from build123d import *

# Parameters (mm, degrees)
CROQUIS1_R              = 4.98
SALIENTE_EXTRUIR1_DEPTH = 4
CROQUIS2_R              = 4.98
SALIENTE_EXTRUIR2_DEPTH = 4
CORTAR_EXTRUIR1_DEPTH   = 12.160680983


with BuildPart() as part:
    # Croquis1 → Saliente-Extruir1 (new body)
    with BuildSketch(Plane(origin=(0, 0, 0), x_dir=(1, 0, 0), z_dir=(0, 1, 0))):
        with Locations(Location((1, 0, 0), (0, 0, 270))):
            Circle(CROQUIS1_R)
    extrude(amount=SALIENTE_EXTRUIR1_DEPTH)

    # Croquis2 → Saliente-Extruir2 (add)
    with BuildSketch(Plane(origin=(0, 4, 0), x_dir=(1, 0, 0), z_dir=(0, 1, 0))):
        with Locations(Location((-1, 0, 0), (0, 0, 78.416067345))):
            Circle(CROQUIS2_R)
    extrude(amount=SALIENTE_EXTRUIR2_DEPTH)

    # Croquis3 → Cortar-Extruir1 (cut, through all)
    with BuildSketch(Plane(origin=(0, 0, 0), x_dir=(1, 0, 0), z_dir=(0, 1, 0))):
        with BuildLine():
            Line((-1.559847749, 2.65), (1.559847749, 2.65))
            ThreePointArc((1.559847749, 2.65), (0, -3.075), (-1.559847749, 2.65))
        make_face()
    extrude(amount=CORTAR_EXTRUIR1_DEPTH, mode=Mode.SUBTRACT)


solid = part.part
Input: part model. Units: mm. Frame: model coordinates. A direction names the side the tool comes from. Round coordinates to 2 decimals unless told otherwise and drop trailing zeros. Loops run counter-clockwise (first coordinate to the right, second up) from the corner with the lowest first, then second, coordinate; pieces in that order, holes last. Notation, with made-up numbers: M 81.5,23 L 89.5,23 A13 cw 89.5,39 Z; hole C -29,74 d8. An arc over 180 degrees is marked long. Answer as CSV lines item,"result". Start each with the question number.
(1) Section B-B, the plane z = 1.5. Output: boundary loops of the cut face in (x, y), plus the area to 3 significant figures.
(2) Reachability of faces 1 (the flat face through (4.3, 4, 0.3)), 2 (the cylindrical face through (2.5, 1.97, 4.75)), 3 (the flat face through (-4.4, 4, 0.1)) from +Z, -Z, +X, -X, +Y, -Y: full face, straight path, thin tool, end or side. Return the list, or none.
(3) Section A-A, the plane x = -2.25. Output: boundary loops of the cut face in (y, z), plus the area to 3 significant figures.
(4) Draft query along Z for faces 4 (the flat face through (0, 4, -2.65)), 5 (the cylindrical face through (-1.512, 5.972, -4.954)), 6 (the flat face through (-3.3, 8, -0.4)). Return one class per face: released by +Z, released by -Z, zero draft, split by the parting line, or undercut.
(5) Section D-D, the plane x = 4.5. Output: boundary loops of the cut face in (y, z), plus the area to 3 significant figures.
(6) First-contact query: pin 1 (5 mm diameter, centred on x = 0, z = 0, fed in from -Y); pin 2 (1.5 mm diameter, centred on y = 3.5, z = 1, fed in from -X); pin 3 (3 mm diameter, centred on x = 4, z = -1.5, fed in from +Y); pin 4 (4 mm diameter, centred on y = 2.5, z = 4, fed in from -X). Flat tips, straight axial feed; report the tip coordinate or a pass-through.
(7) Line query: line 1 (X direction, y = 2, z = 0) (3 decimals); line 2 (X direction, y = 7.75, z = 0) (3 decimals); line 3 (Z direction, x = 0, y = 2) (3 decimals). Output: solid intervals per line, ascending. Write a range as [from, to].
(8) Section C-C, the plane y = 7. Output: boundary loops of the cut face in (x, z) (3 decimals).
Values found:
1,outline,"M -5.75,4 L -3.75,4 L -3.75,0 L -2.68,0 L -2.68,8 L -5.75,8 Z; M 2.68,0 L 5.75,0 L 5.75,4 L 3.75,4 L 3.75,8 L 2.68,8 Z"
1,area,"33.0 mm²"
2,face 1,"+X, +Y"
2,face 2,"-Y"
2,face 3,"-X, -Y"
3,outline,"M 0,-3.77 L 4,-3.77 L 4,-4.82 L 8,-4.82 L 8,-2.1 L 0,-2.1 Z; M 0,2.1 L 8,2.1 L 8,4.82 L 4,4.82 L 4,3.77 L 0,3.77 Z"
3,area,"35.2 mm²"
4,face 4,"undercut"
4,face 5,"split by the parting line"
4,face 6,"zero draft"
5,outline,"M 0,-3.54 L 4,-3.54 L 4,3.54 L 0,3.54 Z"
5,area,"28.3 mm²"
6,pin 1,"passes through"
6,pin 2,"stops at x = -5.96"
6,pin 3,"stops at y = 8"
6,pin 4,"stops at x = -5.2"
7,line 1,"x = [-3.98, -3.075], [3.075, 5.98]"
7,line 2,"x = [-5.98, -3.075], [3.075, 3.98]"
7,line 3,"z = [-4.879, -2.65], [3.075, 4.879]"
8,outline,"C -1,0 d9.96; hole M -1.56,-2.65 L 1.56,-2.65 A3.075 ccw long Z"
